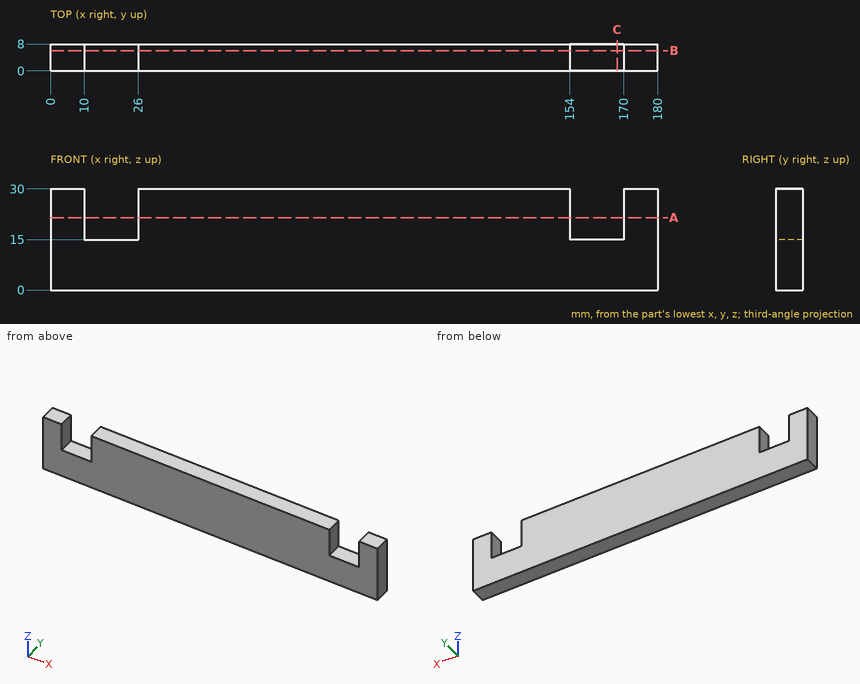
Could you check a few things on this drawing? It's one solid part, dimensions in mm from its lowest x, y, z. Round coordinates to 2 decimals unless told otherwise and drop trailing zeros. Order: outer loops, then holes, each group sorted by start corner. A loop starts at its lowest first (then second) coordinate and runs counter-clockwise, first axis right, second up. Notation, with made-up numbers: M -16.5,6.5 L 3.5,6.5 A21 ccw 3.5,14.5 Z; hole C 38,13.5 d6. An arc over 180 degrees is marked long. One line per item, written item: value.
(1) Imagine slicing it at C-C (x = 168). Write out the boundary of the cut face in (y, z).
Ans:
outline: M 0,0 L 8,0 L 8,15 L 0,15 Z
(2) I'm going to push a flat-ended pin straight in: P1, Ø2.5, axis at x = 15, y = 2.5, coming from the +Z side. Where does the tip first touch, or does it pass through?
Ans:
P1: stops at z = 15
(3) Imagine slicing it at B-B (y = 6). Write out the boundary of the cut face in (x, z).
Ans:
outline: M 0,0 L 180,0 L 180,30 L 170,30 L 170,15 L 154,15 L 154,30 L 26,30 L 26,15 L 10,15 L 10,30 L 0,30 Z
(4) Imagine slicing it at A-A (z = 21.5). Write out the boundary of the cut face in (x, y), and give its area (3 significant figures).
Ans:
outline: M 0,0 L 10,0 L 10,8 L 0,8 Z; M 26,0 L 154,0 L 154,8 L 26,8 Z; M 170,0 L 180,0 L 180,8 L 170,8 Z
area: 1,180 mm^2
(5) I need wall thicknesses on line 1 along X through (y, z) = (5.5, 17.25); line 2 along Z through (x, y) = (163, 6.5). Which ranges of each line are inside material? Lowest first, please. Write a range as from..to.
Ans:
line 1: x = 0..10, 26..154, 170..180
line 2: z = 0..15
